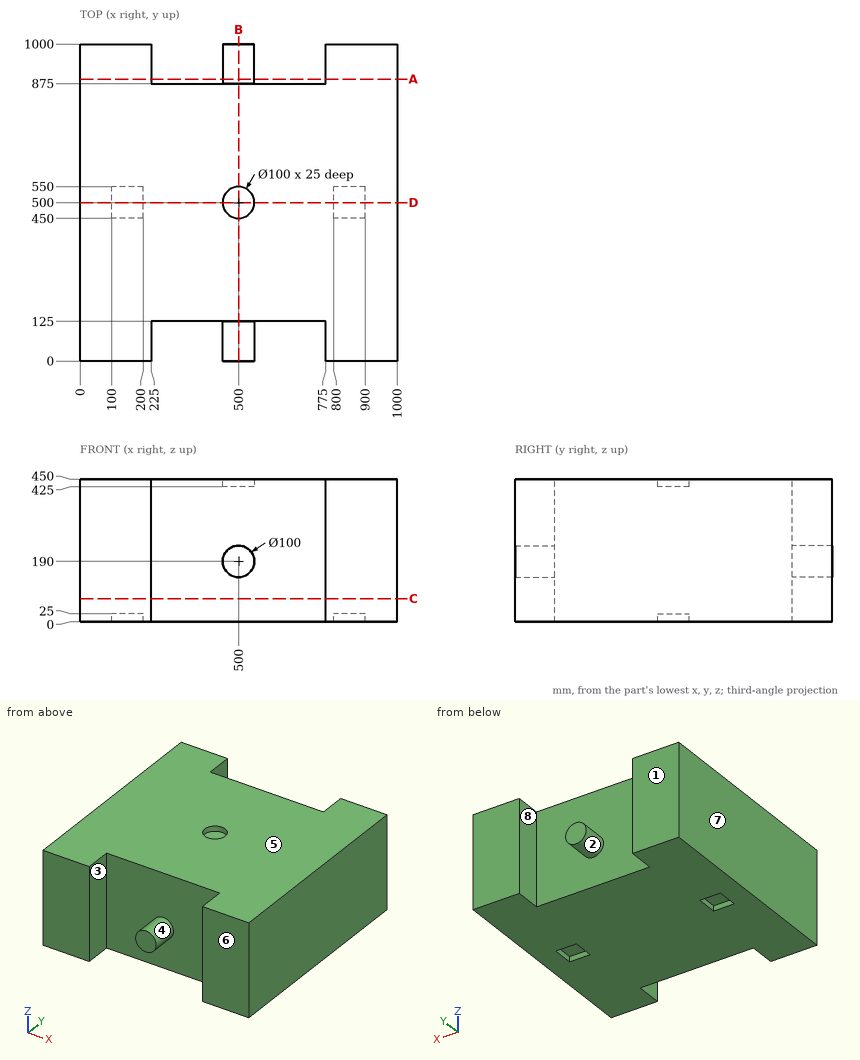
Source: three-view drawing plus pictorial views. Frame: mm from the lowest corner of the part. A direction names the side the tool comes from. Round coordinates to 2 decimals unless told otherwise and drop trailing zeros. Order: outer loops, then holes, each group sorted by start corner. A loop starts at its lowest first (then second) coordinate and runs counter-clockwise, first axis right, second up. Notation, with made-up numbers: (-1.5, 13) -> (10.5, 13) arc R17 ccw to (10.5, 30) -> close; hole circle Ø10 at (46.25, -1.5). An arc over 180 degrees is marked (long way). Use one line per item in the form item = value. Start each with the question number.
1. Pin query (flat end, axial travel): pin 1 Ø4 at (x, z) = (757, 362) entering from -Y; pin 2 Ø6 at (x, z) = (594, 319.5) entering from +Y. Return the tip coordinate at first contact, or that it passes through.
2. Draft query along X for the marked faces 6, 7 and 8. Return one class per face: pulls with the +X half, pulls with the -X half, needs draft (parallel to the pull), parting line crosses it, or undercut.
3. Line query: probe 1 along X at (y, z) = (929, 120.5); probe 2 along Y at (x, z) = (500, 434); probe 3 along Y at (x, z) = (643.5, 248.5). Output: solid intervals per line, ascending.
4. Cut plane B-B (x = 500). Return the cut outline in (y, z), then the cut area to 3 significant figures.
5. Cut plane A-A (y = 889). Return the cut outline in (x, z).
6. Cut plane D-D (y = 500). Return the cut outline in (x, z).
7. Reachability of the marked faces 1, 2, 3, 4 and 5 from +Z, -Z, +X, -X, +Y, -Y: full face, straight path, thin tool, end or side. Return the list, or none.
8. Cut plane C-C (z = 72.5). Return the cut outline in (x, y).
Solution:
q1.pin_1 = 125
q1.pin_2 = 875
q2.face_6 = needs draft
q2.face_7 = pulls with the -X half
q2.face_8 = undercut
q3.probe_1 = 0 to 225, 775 to 1000
q3.probe_2 = 125 to 450, 550 to 875
q3.probe_3 = 125 to 875
q4.outline = (0, 140) -> (125, 140) -> (125, 0) -> (875, 0) -> (875, 140) -> (1000, 140) -> (1000, 240) -> (875, 240) -> (875, 450) -> (550, 450) -> (550, 425) -> (450, 425) -> (450, 450) -> (125, 450) -> (125, 240) -> (0, 240) -> close
q4.area = 360,000 mm^2
q5.outline = (0, 0) -> (225, 0) -> (225, 450) -> (0, 450) -> close; circle Ø100 at (500, 190); (775, 0) -> (1000, 0) -> (1000, 450) -> (775, 450) -> close
q6.outline = (0, 0) -> (100, 0) -> (100, 25) -> (200, 25) -> (200, 0) -> (800, 0) -> (800, 25) -> (900, 25) -> (900, 0) -> (1000, 0) -> (1000, 450) -> (550, 450) -> (550, 425) -> (450, 425) -> (450, 450) -> (0, 450) -> close
q7.face_1 = +Z, -Z, +X, -X, +Y
q7.face_2 = +Y
q7.face_3 = +Z, -Z, -Y
q7.face_4 = -Y
q7.face_5 = +Z, +X, -X, +Y, -Y
q8.outline = (0, 0) -> (225, 0) -> (225, 125) -> (775, 125) -> (775, 0) -> (1000, 0) -> (1000, 1000) -> (775, 1000) -> (775, 875) -> (225, 875) -> (225, 1000) -> (0, 1000) -> close
